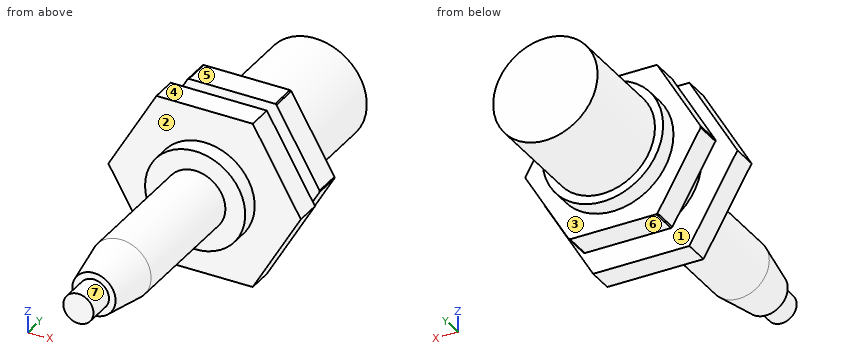
```python
from build123d import *

# Parameters (mm, degrees)
SKETCH2_OUTSIDE_W  = 32.818
SKETCH2_OUTSIDE_H  = 32.818
CUT_EXTRUDE1_DEPTH = 2.667
CHAMFER1_SIZE      = 5.08
CHAMFER1_SIZE2     = 0.895741062
SKETCH3_OUTSIDE_W  = 32.684
SKETCH3_OUTSIDE_H  = 30.854
CUT_EXTRUDE2_DEPTH = 2.794
CUT_EXTRUDE3_START = 2.5
CUT_EXTRUDE3_DEPTH = 2.5


with BuildPart() as part:
    # Sketch1 → Revolve1 (revolve)
    with BuildSketch(Plane.XY, mode=Mode.PRIVATE) as revolve1_sk:
        Polygon((1.5875, -26.416), (1.5875, -23.495), (3.175, -23.495), (3.175, -4.445), (5.2705, -4.445), (5.2705, -2.667), (10.1219, -2.667), (10.1219, 0), (6.35, 0), (6.35, 2.5), (9.2075, 2.5), (9.2075, 5.294), (6.35, 5.294), (6.35, 7.239), (5.49275, 7.239), (5.49275, 18.034), (0, 18.034), (0, -26.416), align=None)
    revolve(revolve1_sk.sketch.rotate(Axis((0, 42.258635304, 0), (0, -1, 0)), 180), axis=Axis((0, 42.258635304, 0), (0, -1, 0)))

    # Sketch2 outside → Cut-Extrude1 (cut)
    with BuildSketch(Plane.XZ.offset(2.667)):
        Rectangle(SKETCH2_OUTSIDE_W, SKETCH2_OUTSIDE_H)
        Polygon((-5.06095, 8.765822535), (5.06095, 8.765822535), (10.1219, 0), (5.06095, -8.765822535), (-5.06095, -8.765822535), (-10.1219, 0), align=None, mode=Mode.SUBTRACT)
    extrude(amount=-CUT_EXTRUDE1_DEPTH, mode=Mode.SUBTRACT)

    # Chamfer1
    chamfer1_edges = [part.edges().sort_by_distance(p)[0] for p in [
        (3.175, -23.495, 0),
    ]]
    chamfer1_side = [part.faces().sort_by_distance(p)[0] for p in [
        (3.175, -13.97, 0),
    ]]
    chamfer(chamfer1_edges, length=CHAMFER1_SIZE, length2=CHAMFER1_SIZE2, reference=chamfer1_side[0])

    # Sketch3 outside → Cut-Extrude2 (cut)
    with BuildSketch(Plane(origin=(0, 5.294, 0), x_dir=(1, 0, 0), z_dir=(0, 1, 0))):
        Rectangle(SKETCH3_OUTSIDE_W, SKETCH3_OUTSIDE_H)
        Polygon((4.626711852, -8.0137), (9.253423704, 0), (4.626711852, 8.0137), (-4.626711852, 8.0137), (-9.253423704, 0), (-4.626711852, -8.0137), align=None, mode=Mode.SUBTRACT)
    extrude(amount=-CUT_EXTRUDE2_DEPTH, mode=Mode.SUBTRACT)

    # Sketch4 → Cut-Extrude3 (cut)
    with BuildSketch(Plane(origin=(0, 0, 0), x_dir=(1, 0, 0), z_dir=(0, 1, 0)).offset(CUT_EXTRUDE3_START)):
        with BuildLine():
            Line((-3.341032774, 5.4), (3.341032774, 5.4))
            ThreePointArc((3.341032774, 5.4), (0, 6.35), (-3.341032774, 5.4))
        make_face()
    extrude(amount=-CUT_EXTRUDE3_DEPTH, mode=Mode.SUBTRACT)


solid = part.part
```
Here's how the part is built. I have some questions about the finished solid (model axes, mm). Face numbers are marked on the shaded views. A direction names the side the tool comes from. Coordinates: 2 decimals unless noted, no trailing zeros. Order: outer loops, then holes, each group sorted by start corner. A loop starts at its lowest first (then second) coordinate and runs counter-clockwise, first axis right, second up. Notation, with made-up numbers: (-28.5, -13.75) - (23.5, -13.75) arc R14 ccw to (23.5, 6.25) - close; hole circle Ø2 at (66.5, 81). An arc over 180 degrees is marked (long way). One line per question, with ' | ' between items.
(1) For the marked faces 5, 6 and 7, which set-ups out of +Z, -Z, +X, -X, +Y, -Y let a thin tool reach every point of the face, with its end or its side?
Report:
face 5: +Z, +X, -X, +Y | face 6: -Z, +X, -X, +Y | face 7: -Y
(2) If we mould it in two halves opening along Y, with no side actions, what happens to the marked faces 1, 2, 3 and 4? For each: pulls with the +Y half, pulls with the -Y half, needs draft (parallel to the pull), parting line crosses it, or undercut.
Report:
face 1: undercut | face 2: pulls with the -Y half | face 3: pulls with the +Y half | face 4: needs draft
(3) Suppose I cut it at A-A on x = -7.25. List the corners of the cut face in (y, z) for me.
Report:
outline: (-2.67, -4.97) - (0, -4.97) - (0, 4.97) - (-2.67, 4.97) - close; (2.5, -3.47) - (5.29, -3.47) - (5.29, 3.47) - (2.5, 3.47) - close
(4) Suppose I cut it at D-D on y = -2. List the corners of the cut face in (x, z) for me.
Report:
outline: (-10.12, 0) - (-5.06, -8.77) - (5.06, -8.77) - (10.12, 0) - (5.06, 8.77) - (-5.06, 8.77) - close
(5) If I drill on L1, parallel to Y at x = 1.75, z = -7.5; L2, parallel to Y at x = -2.5, z = -5.75; L3, parallel to Y at x = 8, z = 2.75, over which ranges is the centre line in solid material (lowest first)?
Report:
L1: y = -2.67 to 0, 2.5 to 5.29 | L2: y = -2.67 to 0, 2.5 to 7.24 | L3: y = -2.67 to 0
(6) Suppose I cut it at C-C on z = 3.75. List the corners of the cut face in (x, y) for me (3 decimals), and give its area (3 significant figures).
Report:
outline: (-7.957, -2.667) - (-3.703, -2.667) - (-3.703, -4.445) - (3.703, -4.445) - (3.703, -2.667) - (7.957, -2.667) - (7.957, 0) - (5.124, 0) - (5.124, 2.5) - (7.088, 2.5) - (7.088, 5.294) - (5.124, 5.294) - (5.124, 7.239) - (4.013, 7.239) - (4.013, 18.034) - (-4.013, 18.034) - (-4.013, 7.239) - (-5.124, 7.239) - (-5.124, 5.294) - (-7.088, 5.294) - (-7.088, 2.5) - (-5.124, 2.5) - (-5.124, 0) - (-7.957, 0) - close | area: 227 mm2
(7) Will these pins go through, and if not, where does the flat tip stop? pin 1 (2 mm diameter, centred on y = -9.5, z = -1, fed in from +X) (3 decimals); pin 2 (4 mm diameter, centred on y = -12, z = 1, fed in from -X) (3 decimals); pin 3 (10 mm diameter, centred on y = -3.5, z = 6, fed in from +X); pin 4 (1.5 mm diameter, centred on y = -14.5, z = 5, fed in from -X).
Report:
pin 1: stops at x = 3.175 | pin 2: stops at x = -3.175 | pin 3: stops at x = 9.5 | pin 4: passes through
